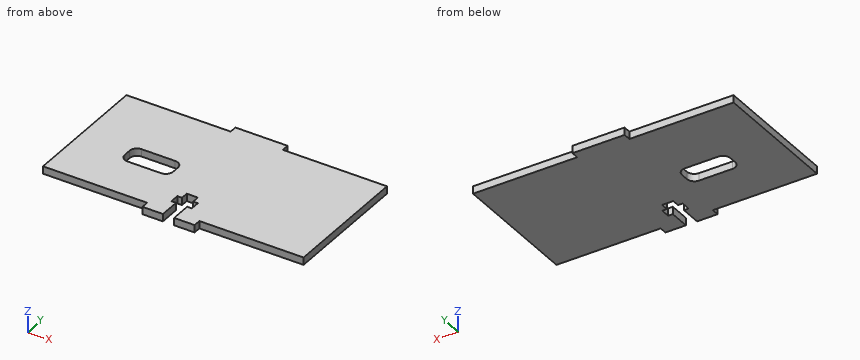
```python
from build123d import *

# Parameters (mm, degrees)
SKETCH1_W                   = 13
SKETCH1_H                   = 6
MAIN_SLIDER_SIDE_UP_DEPTH   = 2
SLIDER_SIDE_UP_CONTOURING_R = 2


with BuildPart() as part:
    # Sketch1 → Main Slider Side Up (new body)
    with BuildSketch(Plane.XY):
        Polygon((42, 35), (70, 35), (70, 0), (42, 0), (42, -2), (36.5, -2), (36.5, 3.5), (37.75, 3.5), (37.75, 6), (36.5, 6), (36.5, 8), (33.5, 8), (33.5, 6), (32.25, 6), (32.25, 3.5), (33.5, 3.5), (33.5, -2), (28, -2), (28, 0), (0, 0), (0, 35), (28, 35), (28, 37), (42, 37), align=None)
        with Locations((19.5, 15)):
            Rectangle(SKETCH1_W, SKETCH1_H, mode=Mode.SUBTRACT)
    extrude(amount=MAIN_SLIDER_SIDE_UP_DEPTH)

    # Slider Side Up Contouring
    slider_side_up_contouring_edges = [part.edges().sort_by_distance(p)[0] for p in [
        (26, 12, 1),
        (26, 18, 1),
        (13, 18, 1),
        (13, 12, 1),
    ]]
    fillet(slider_side_up_contouring_edges, radius=SLIDER_SIDE_UP_CONTOURING_R)


solid = part.part
```
The listing builds one solid part. Answer for the finished solid, in the listing's coordinates (mm). Give positions to 0.01 mm unless a question says otherwise; leave off trailing zeros. Loops run counter-clockwise (first coordinate to the right, second up) from the corner with the lowest first, then second, coordinate; pieces in that order, holes last. Notation, with made-up numbers: M -19,-7.5 L 8,-7.5 A29 cw 8,20.5 Z; hole C -38,24 d9. An arc over 180 degrees is marked long. One line per item, written item: value.
Q1. A cutting plane is placed at D-D on x = 56. Determine the outline of the cut face in (y, z), then the cut area to 3 significant figures.
Working result:
outline: M 0,0 L 35,0 L 35,2 L 0,2 Z
area: 70.0 mm^2
Q2. Find the intervals of material crossed by line 1 (Y direction, x = 22, z = 1.4); line 2 (X direction, y = 14.5, z = 1.7); line 3 (X direction, y = 0.5, z = 1.2), in increasing order. Write a range as from..to.
Working result:
line 1: y = 0..12, 18..35
line 2: x = 0..13, 26..70
line 3: x = 0..33.5, 36.5..70
Q3. A cutting plane is placed at C-C on x = 35.5. Determine the outline of the cut face in (y, z), then the cut area to 3 significant figures.
Working result:
outline: M 8,0 L 37,0 L 37,2 L 8,2 Z
area: 58.0 mm^2
Q4. A cutting plane is placed at A-A on x = 19. Determine the outline of the cut face in (y, z).
Working result:
outline: M 0,0 L 12,0 L 12,2 L 0,2 Z; M 18,0 L 35,0 L 35,2 L 18,2 Z
Q5. Flat-ended cylindrical pins translate along their axes: P1, Ø12, axis at x = 13, y = 22.5, coming from the -Z side; P2, Ø0.6, axis at x = 55, z = 0.5, coming from the -Y side; P3, Ø0.6, axis at x = 21, z = 1, coming from the +Y side. Find the tip coordinate at first contact, or state that the pin passes through.
Working result:
P1: stops at z = 0
P2: stops at y = 0
P3: stops at y = 35
